Here's the drawing with two shaded views (mm, measured from the low corner). I have some questions. Coordinates: 2 decimals unless noted, no trailing zeros. Write each loop counter-clockwise with the first axis right and the second up, starting at its lowest first coordinate (ties: lowest second). Pieces come first, ordered by that corner, then holes. Notation, with made-up numbers: M 50,77 L 99,77 A26 cw 99,105 Z; hole C 61,43 d8. An arc over 180 degrees is marked long. Use one line per item in the form item = value. Start each with the question number.
1. Please list where these lines run through material, in increasing order: line 1 along X through (y, z) = (8.5, 14); line 2 along X through (y, z) = (1.7, 4); line 3 along Z through (x, y) = (83, 0.75). Write a range as [from, to].
2. I want a section at A-A, the plane x = 4. List the corners of the cut face in (y, z) for me.
3. Thinking about a two-plate mould opening in Z: for the marked faces 1, 2 and 3, which applies, released by +Z, released by -Z, zero draft, split by the parting line, or undercut?
4. I want a section at B-B, the plane y = 9. List the corners of the cut face in (x, z) for me.
5. I want a section at D-D, the plane z = 4. List the corners of the cut face in (x, y) for me.
6. I want a section at C-C, the plane x = 83. List the corners of the cut face in (y, z) for me.
7. I'm going to push flat-ended pins straight in: pin 1 Ø3 at (x, z) = (16, 59) entering from -Y; pin 2 Ø12 at (x, z) = (88, 28.5) entering from -Y; pin 3 Ø3 at (x, z) = (15.5, 20) entering from +Y. Where does each tip first touch, or does it pass through?
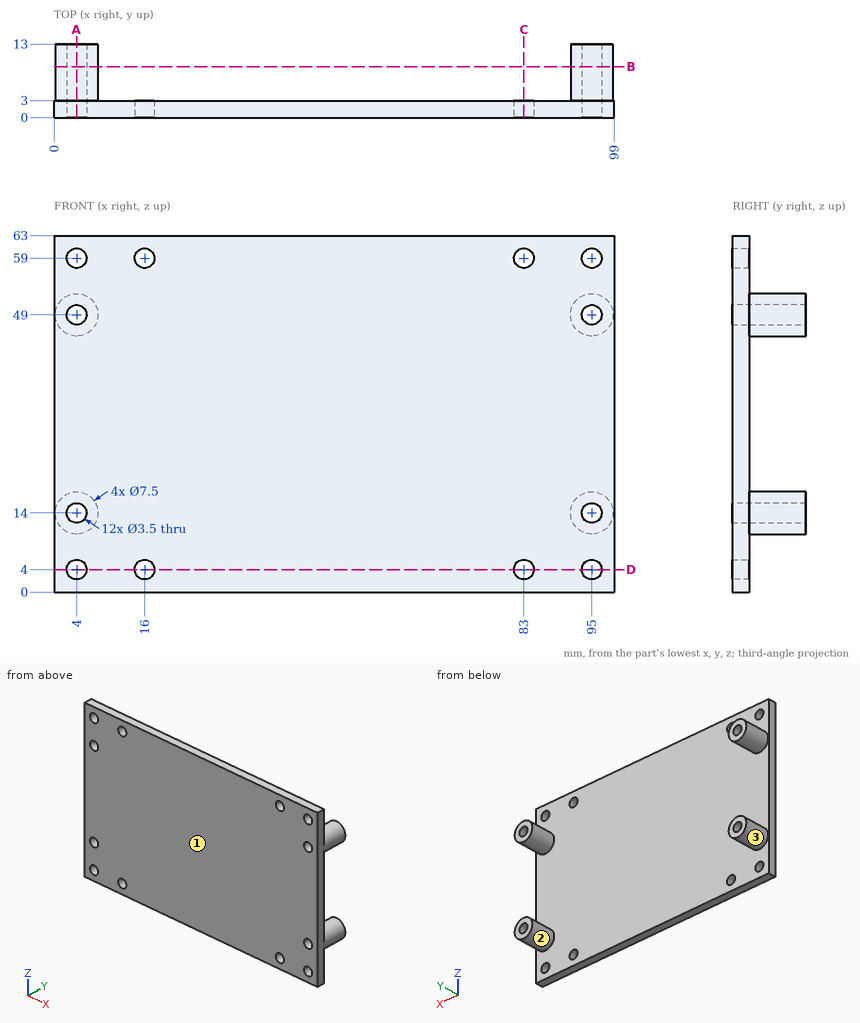
Answer list:
q1.line_1 = [0.25, 2.25], [5.75, 7.75], [91.25, 93.25], [96.75, 98.75]
q1.line_2 = [0, 2.25], [5.75, 14.25], [17.75, 81.25], [84.75, 93.25], [96.75, 99]
q1.line_3 = [0, 2.25], [5.75, 57.25], [60.75, 63]
q2.outline = M 0,0 L 3,0 L 3,2.25 L 0,2.25 Z; M 0,5.75 L 3,5.75 L 3,10.25 L 13,10.25 L 13,12.25 L 0,12.25 Z; M 0,15.75 L 13,15.75 L 13,17.75 L 3,17.75 L 3,45.25 L 13,45.25 L 13,47.25 L 0,47.25 Z; M 0,50.75 L 13,50.75 L 13,52.75 L 3,52.75 L 3,57.25 L 0,57.25 Z; M 0,60.75 L 3,60.75 L 3,63 L 0,63 Z
q3.face_1 = zero draft
q3.face_2 = undercut
q3.face_3 = undercut
q4.outline = C 4,14 d7.5; C 4,49 d7.5; C 95,14 d7.5; C 95,49 d7.5; hole C 4,14 d3.5; hole C 4,49 d3.5; hole C 95,14 d3.5; hole C 95,49 d3.5
q5.outline = M 0,0 L 2.25,0 L 2.25,3 L 0,3 Z; M 5.75,0 L 14.25,0 L 14.25,3 L 5.75,3 Z; M 17.75,0 L 81.25,0 L 81.25,3 L 17.75,3 Z; M 84.75,0 L 93.25,0 L 93.25,3 L 84.75,3 Z; M 96.75,0 L 99,0 L 99,3 L 96.75,3 Z
q6.outline = M 0,0 L 3,0 L 3,2.25 L 0,2.25 Z; M 0,5.75 L 3,5.75 L 3,57.25 L 0,57.25 Z; M 0,60.75 L 3,60.75 L 3,63 L 0,63 Z
q7.pin_1 = through
q7.pin_2 = 0
q7.pin_3 = 3
